```python
from build123d import *

# Parameters (mm, degrees)
F1_DEPTH = 19.05
F2_DEPTH = 9.525


with BuildPart() as f1:
    # F0 (on Right) → F1 (new body)
    with BuildSketch(Plane.YZ):
        Polygon((-42.835101, 79.173712), (-50.772601, 79.173712), (-50.772601, -143.076288), (-41.234901, -143.076288), (-41.234901, -124.026288), (-34.122901, -124.026288), (-27.010901, -124.026288), (-27.010901, -143.076288), (-17.473201, -143.076288), (-17.473201, 79.173712), (-25.410701, 79.173712), (-25.410701, 60.123712), (-34.122901, 60.123712), (-42.835101, 60.123712), align=None)
    extrude(amount=F1_DEPTH)

    # F0 (on Right) → F2 (join)
    with BuildSketch(Plane.YZ):
        Polygon((-42.835101, 79.173712), (-50.772601, 79.173712), (-50.772601, -143.076288), (-41.234901, -143.076288), (-41.234901, -124.026288), (-34.122901, -124.026288), (-27.010901, -124.026288), (-27.010901, -143.076288), (-17.473201, -143.076288), (-17.473201, 79.173712), (-25.410701, 79.173712), (-25.410701, 60.123712), (-34.122901, 60.123712), (-42.835101, 60.123712), align=None)
    extrude(amount=F2_DEPTH)


solid = f1.part
```
For this review, take the finished solid that the model builds, in its own axes (mm). A direction names the side the tool comes from. Give positions to 0.01 mm unless a question says otherwise; leave off trailing zeros. Write each loop counter-clockwise with the first axis right and the second up, starting at its lowest first coordinate (ties: lowest second). Pieces come first, ordered by that corner, then holes. Notation, with made-up numbers: M -35.5,8.5 L 20.5,8.5 A7 ccw 20.5,17.5 Z; hole C 66,-37 d11. An arc over 180 degrees is marked long. Answer as CSV lines item,"result".
1. For pin 1 (7 mm diameter, centred on x = 11, y = -31.5, fed in from -Z); pin 2 (5 mm diameter, centred on x = 10.5, y = -39.5, fed in from +Z), all flat-tipped, find the tip position at first contact; note any pin that passes through.
Findings:
pin 1,"stops at z = -124.03"
pin 2,"stops at z = 60.12"
2. Consider section B-B, the plane y = -33.5. Write out the cut boundary in (x, z).
Findings:
outline,"M 0,-124.03 L 19.05,-124.03 L 19.05,60.12 L 0,60.12 Z"
3. For faces 4 (the flat face through (9, -34, -124.026)), 5 (the flat face through (9, -42.835, 70)), 6 (the flat face through (9, -17.473, -34)), list the 3-axis set-ups (+Z, -Z, +X, -X, +Y, -Y) from which the entire face can be reached by the end or side of a thin tool; tool diameter is ignored.
Findings:
face 4,"-Z, +X, -X"
face 5,"+Z, +X, -X"
face 6,"+Z, -Z, +X, -X, +Y"
4. Draft analysis for pull direction Y (two halves, no side actions). For faces 1 (the flat face through (9, -41.235, -134)), 2 (the flat face through (9, -50.773, -30)), 3 (the flat face through (9, -21, 79.174)), state which applies: +Y half, -Y half, draft (parallel to the pull), parting line (faces both ways), or undercut.
Findings:
face 1,"undercut"
face 2,"-Y half"
face 3,"draft"
5. Wall thickness on line 1 (Y direction, x = 13.75, z = -128.5); line 2 (Y direction, x = 11.25, z = 61); line 3 (Z direction, x = 15.75, y = -40): over which ranges is each line inside the solid? List them lowest first.
Findings:
line 1,"y = -50.77 to -41.23, -27.01 to -17.47"
line 2,"y = -50.77 to -42.84, -25.41 to -17.47"
line 3,"z = -124.03 to 60.12"
6. Consider section A-A, the plane x = 17. Write out the cut boundary in (y, z).
Findings:
outline,"M -50.77,-143.08 L -41.23,-143.08 L -41.23,-124.03 L -27.01,-124.03 L -27.01,-143.08 L -17.47,-143.08 L -17.47,79.17 L -25.41,79.17 L -25.41,60.12 L -42.84,60.12 L -42.84,79.17 L -50.77,79.17 Z"
